from build123d import *

# Parameters (mm, degrees)
SKETCH1_R               = 75
SKETCH1_R_2             = 5
BOSS_EXTRUDE1_DEPTH     = 10
SKETCH4_R               = 1.5
CUT_EXTRUDE1_DEPTH      = 1
CUT_EXTRUDE1_DEPTH_BACK = 11


with BuildPart() as part:
    # Sketch1 → Boss-Extrude1 (new body)
    with BuildSketch(Plane(origin=(0, 0, 0), x_dir=(1, 0, 0), z_dir=(0, 1, 0))):
        Circle(SKETCH1_R)
        Circle(SKETCH1_R_2, mode=Mode.SUBTRACT)
    extrude(amount=BOSS_EXTRUDE1_DEPTH)

    # Sketch4 → Cut-Extrude1 (cut, two sides)
    with BuildSketch(Plane(origin=(0, 10, 0), x_dir=(1, 0, 0), z_dir=(0, 1, 0))) as cut_extrude1_sk:
        with Locations((-26.550808926, -53.805711085)):
            Circle(SKETCH4_R)
        with Locations((-30.975943747, -62.773329599)):
            Circle(SKETCH4_R)
        with Locations((-63.01509769, 30.480268572)):
            Circle(SKETCH4_R)
        with Locations((-54.047479176, 26.05513375)):
            Circle(SKETCH4_R)
        with Locations((62.277654423, -30.734175657)):
            Circle(SKETCH4_R)
        with Locations((53.310035909, -26.309040836)):
            Circle(SKETCH4_R)
        with Locations((-4.853556436, 69.978752855)):
            Circle(SKETCH4_R)
        with Locations((-4.202026349, 60)):
            Circle(SKETCH4_R)
        with Locations((49.896530564, 33.321708205)):
            Circle(SKETCH4_R)
        with Locations((58.212618991, 38.875326239)):
            Circle(SKETCH4_R)
    extrude(amount=CUT_EXTRUDE1_DEPTH, mode=Mode.SUBTRACT)
    extrude(cut_extrude1_sk.sketch, amount=-CUT_EXTRUDE1_DEPTH_BACK, mode=Mode.SUBTRACT)


solid = part.part
Work out the finished part from the listing and answer in its coordinate system (mm). Round coordinates to 2 decimals unless told otherwise and drop trailing zeros. Loops run counter-clockwise (first coordinate to the right, second up) from the corner with the lowest first, then second, coordinate; pieces in that order, holes last. Notation, with made-up numbers: M -8,2 L -4,2 A22 ccw -4,29 Z; hole C 4,-2.5 d6. An arc over 180 degrees is marked long. One line per question, with ' | ' between items. Start each with the question number.
(1) A cutting plane is placed at A-A on z = 0. Write down the section's boundary in (x, y), plus the area to 3 significant figures.
(2) A cutting plane is placed at B-B on x = 0. Write down the section's boundary in (y, z), plus the area to 3 significant figures.
(3) Find the intervals of material crossed by line 1 (X direction, y = 4, z = -4); line 2 (Z direction, x = -31, y = 7.75); line 3 (Z direction, x = -26.5, y = 8), in increasing order.
(4) Flat-ended cylindrical pins translate along their axes: pin 1 Ø1.5 at (y, z) = (6, -20) entering from -X; pin 2 Ø6 at (x, y) = (51.5, 6.5) entering from -Z; pin 3 Ø4 at (y, z) = (4, 11) entering from +X. Find the tip coordinate at first contact, or state that the pin passes through.
(5) A cutting plane is placed at D-D on x = 28. Write down the section's boundary in (y, z), plus the area to 3 significant figures.
(6) A cutting plane is placed at C-C on y = 6.5. Give the number of separate pieces and of enclosed holes in the cut face, plus the area to 3 significant figures.
(7) For a pull along X with two mould halves and no side action, classify faces 1 (the face through (-9.764, 4.93, -74.362)), 2 (the face through (-1, 10, 16)), 3 (the face through (-1.08, 4.93, 4.88)) as released by +X, released by -X, zero draft, split by the parting line, or undercut.
Geometry check:
1) outline: M -75,0 L -5,0 L -5,10 L -75,10 Z; M 5,0 L 75,0 L 75,10 L 5,10 Z | area: 1,400 mm²
2) outline: M 0,-75 L 10,-75 L 10,-5 L 0,-5 Z; M 0,5 L 10,5 L 10,75 L 0,75 Z | area: 1,400 mm²
3) line 1: x = -74.89 to -3, 3 to 74.89 | line 2: z = -68.29 to 61.27, 64.27 to 68.29 | line 3: z = -70.16 to 52.31, 55.3 to 70.16
4) pin 1: stops at x = -72.49 | pin 2: stops at z = -57.21 | pin 3: stops at x = 74.46
5) outline: M 0,-69.58 L 10,-69.58 L 10,69.58 L 0,69.58 Z | area: 1,390 mm²
6) separate pieces: 1 | enclosed holes: 11 | area: 17,500 mm²
7) face 1: split by the parting line | face 2: zero draft | face 3: undercut
